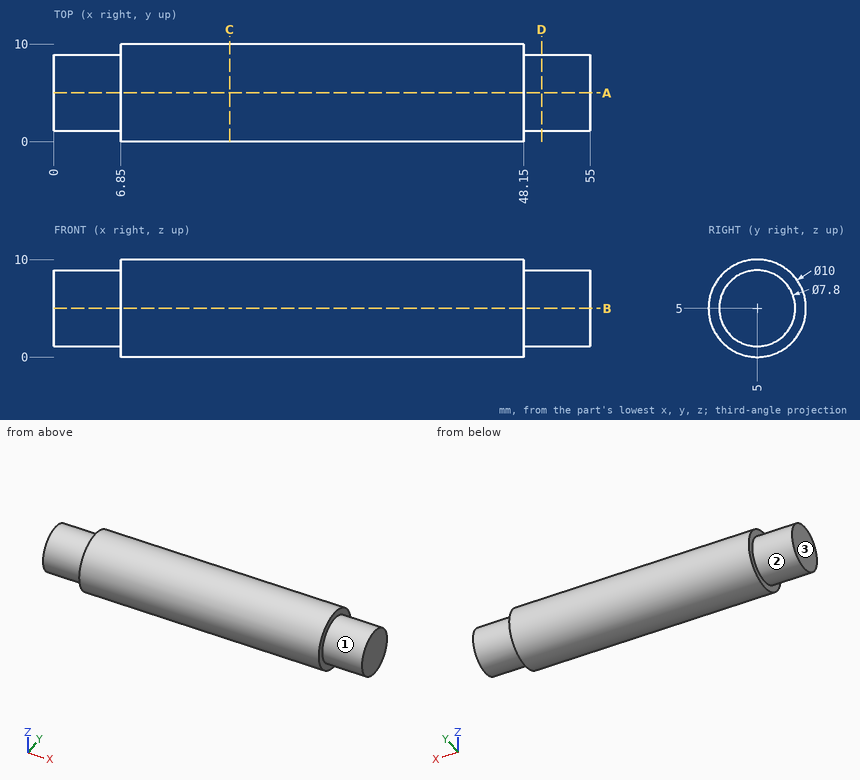
Here's the drawing with two shaded views (mm, measured from the low corner). I have some questions. A direction names the side the tool comes from. Give positions to 0.01 mm unless a question says otherwise; leave off trailing zeros. Loops run counter-clockwise (first coordinate to the right, second up) from the corner with the lowest first, then second, coordinate; pieces in that order, holes last. Notation, with made-up numbers: (58.25, 88) -> (92.25, 88) arc R19 ccw to (92.25, 106) -> close; hole circle Ø2 at (53.25, 3.25). An arc over 180 degrees is marked (long way). Answer as a JSON object with one key per item and string values. Group by question number.
Item 1: Imagine slicing it at A-A on y = 5. Write out the boundary of the cut face in (x, z).
Item 2: Imagine slicing it at C-C on x = 18. Write out the boundary of the cut face in (y, z), then the cut area to 3 significant figures.
Item 3: On a 3-axis mill with a long thin cutter (end or side, diameter ignored), from which of +Z, -Z, +X, -X, +Y, -Y can I reach the whole of each face in a straight line? I mean the marked faces 1, 2 and 3. Say none if no direction works.
Item 4: I need wall thicknesses on L1, parallel to X at y = 3, z = 1; L2, parallel to Z at x = 8.5, y = 4.25; L3, parallel to Z at x = 27, y = 6.5. Which ranges of each line are inside material? Lowest first, please.
Item 5: Will these pins go through, and if not, where does the flat tip stop? pin 1 (1 mm diameter, centred on x = 13, z = 6.5, fed in from -Y); pin 2 (4 mm diameter, centred on y = 3, z = 5, fed in from -X); pin 3 (2 mm diameter, centred on x = 29, z = 6.5, fed in from +Y); pin 4 (5 mm diameter, centred on x = 14, y = 8, fed in from -Z).
Item 6: Imagine slicing it at D-D on x = 50. Write out the boundary of the cut face in (y, z), then the cut area to 3 significant figures.
Answer list:
{
 "1": {"outline": "(0, 1.1) -> (6.85, 1.1) -> (6.85, 0) -> (48.15, 0) -> (48.15, 1.1) -> (55, 1.1) -> (55, 8.9) -> (48.15, 8.9) -> (48.15, 10) -> (6.85, 10) -> (6.85, 8.9) -> (0, 8.9) -> close"},
 "2": {"outline": "circle Ø10 at (5, 5)", "area": "78.5 mm2"},
 "3": {"face 1": "+X", "face 2": "-X", "face 3": "+Z, -Z, -X, +Y, -Y"},
 "4": {"L1": "x = 6.85 to 48.15", "L2": "z = 0.06 to 9.94", "L3": "z = 0.23 to 9.77"},
 "5": {"pin 1": "stops at y = 0.1", "pin 2": "stops at x = 0", "pin 3": "stops at y = 9.97", "pin 4": "stops at z = 0.03"},
 "6": {"outline": "circle Ø7.8 at (5, 5)", "area": "47.8 mm2"}
}
